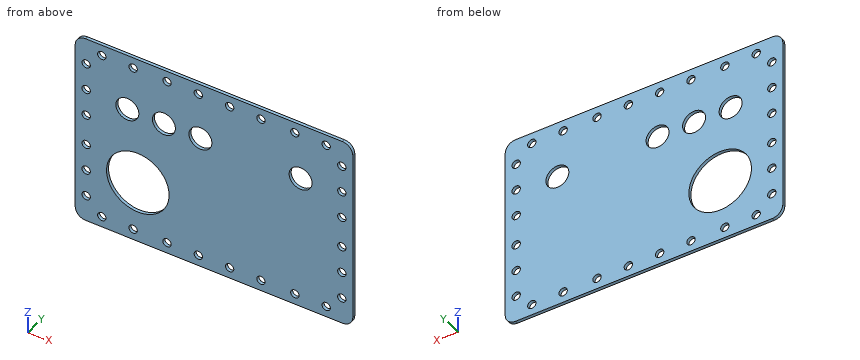
from build123d import *

# Parameters (mm, degrees)
SKETCH1_W           = 266
SKETCH1_H           = 186
BOSS_EXTRUDE1_DEPTH = 3
FILLET1_R           = 10
SKETCH2_R           = 4
SKETCH2_R_2         = 30
SKETCH2_R_3         = 11
CUT_EXTRUDE1_DEPTH  = 163.317589928


with BuildPart() as part:
    # Sketch1 → Boss-Extrude1 (new body)
    with BuildSketch(Plane(origin=(0, 0, 0), x_dir=(1, 0, 0), z_dir=(0, 1, 0))):
        Rectangle(SKETCH1_W, SKETCH1_H)
    extrude(amount=BOSS_EXTRUDE1_DEPTH)

    # Fillet1
    fillet1_edges = [part.edges().sort_by_distance(p)[0] for p in [
        (-133, 1.5, -93),
        (133, 1.5, -93),
        (133, 1.5, 93),
        (-133, 1.5, 93),
    ]]
    fillet(fillet1_edges, radius=FILLET1_R)

    # Sketch2 → Cut-Extrude1 (cut, through all)
    with BuildSketch(Plane(origin=(0, 3, 0), x_dir=(1, 0, 0), z_dir=(0, 1, 0))):
        with Locations(Location((-122.5, -15, 0), (0, 0, 270))):
            Circle(SKETCH2_R)
        with Locations(Location((-122.5, -41.25, 0), (0, 0, 270))):
            Circle(SKETCH2_R)
        with Locations(Location((-122.5, -67.5, 0), (0, 0, 270))):
            Circle(SKETCH2_R)
        with Locations(Location((-107.5, -82.5, 0), (0, 0, 270))):
            Circle(SKETCH2_R)
        with Locations(Location((-77.5, -82.5, 0), (0, 0, 270))):
            Circle(SKETCH2_R)
        with Locations(Location((-45, -82.5, 0), (0, 0, 270))):
            Circle(SKETCH2_R)
        with Locations(Location((-15, -82.5, 0), (0, 0, 270))):
            Circle(SKETCH2_R)
        with Locations(Location((-15, 82.5, 0), (0, 0, 90))):
            Circle(SKETCH2_R)
        with Locations(Location((-45, 82.5, 0), (0, 0, 90))):
            Circle(SKETCH2_R)
        with Locations(Location((-77.5, 82.5, 0), (0, 0, 90))):
            Circle(SKETCH2_R)
        with Locations(Location((-107.5, 82.5, 0), (0, 0, 90))):
            Circle(SKETCH2_R)
        with Locations(Location((-122.5, 67.5, 0), (0, 0, 90))):
            Circle(SKETCH2_R)
        with Locations(Location((-122.5, 41.25, 0), (0, 0, 90))):
            Circle(SKETCH2_R)
        with Locations(Location((-122.5, 15, 0), (0, 0, 90))):
            Circle(SKETCH2_R)
        with Locations(Location((15, -82.5, 0), (0, 0, 90))):
            Circle(SKETCH2_R)
        with Locations(Location((107.5, -82.5, 0), (0, 0, 90))):
            Circle(SKETCH2_R)
        with Locations(Location((122.5, -67.5, 0), (0, 0, 90))):
            Circle(SKETCH2_R)
        with Locations(Location((122.5, -41.25, 0), (0, 0, 90))):
            Circle(SKETCH2_R)
        with Locations(Location((122.5, -15, 0), (0, 0, 90))):
            Circle(SKETCH2_R)
        with Locations(Location((122.5, 15, 0), (0, 0, 270))):
            Circle(SKETCH2_R)
        with Locations(Location((122.5, 41.25, 0), (0, 0, 270))):
            Circle(SKETCH2_R)
        with Locations(Location((122.5, 67.5, 0), (0, 0, 270))):
            Circle(SKETCH2_R)
        with Locations(Location((107.5, 82.5, 0), (0, 0, 270))):
            Circle(SKETCH2_R)
        with Locations(Location((77.5, 82.5, 0), (0, 0, 270))):
            Circle(SKETCH2_R)
        with Locations(Location((45, 82.5, 0), (0, 0, 270))):
            Circle(SKETCH2_R)
        with Locations(Location((15, 82.5, 0), (0, 0, 270))):
            Circle(SKETCH2_R)
        with Locations(Location((-73, 33, 0), (0, 0, 270))):
            Circle(SKETCH2_R_2)
        with Locations(Location((83, -38, 0), (0, 0, 270))):
            Circle(SKETCH2_R_3)
        with Locations(Location((-83, -38, 0), (0, 0, 270))):
            Circle(SKETCH2_R_3)
        with Locations(Location((-48, -38, 0), (0, 0, 270))):
            Circle(SKETCH2_R_3)
        with Locations(Location((-13, -38, 0), (0, 0, 270))):
            Circle(SKETCH2_R_3)
        with Locations(Location((45, -82.5, 0), (0, 0, 90))):
            Circle(SKETCH2_R)
        with Locations(Location((77.5, -82.5, 0), (0, 0, 90))):
            Circle(SKETCH2_R)
    extrude(amount=-CUT_EXTRUDE1_DEPTH, mode=Mode.SUBTRACT)


solid = part.part
Geometry check sheet. Reference: the model listing, model coordinates, mm. Round coordinates to 2 decimals unless told otherwise and drop trailing zeros. Write each loop counter-clockwise with the first axis right and the second up, starting at its lowest first coordinate (ties: lowest second). Pieces come first, ordered by that corner, then holes.
Item 1: Go/stop test with flat-tipped pins: pin 1 Ø13 at (x, z) = (-15, -82.5) entering from -Y; pin 2 Ø5 at (x, z) = (-122.5, -67.5) entering from +Y. Record where each tip stops, or that it passes through.
Determined:
pin 1: stops at y = 0
pin 2: passes through
Item 2: Section check D-D (y = 1.1). Give the number of separate pieces and of enclosed holes in the cut face, plus the area to 3 significant figures.
Determined:
separate pieces: 1
enclosed holes: 33
area: 43,600 mm2
Item 3: Section check A-A (x = 15). Record the boundary of the cut face in (y, z).
Determined:
outline: (0, -93) - (3, -93) - (3, -86.5) - (0, -86.5) - close; (0, -78.5) - (3, -78.5) - (3, 78.5) - (0, 78.5) - close; (0, 86.5) - (3, 86.5) - (3, 93) - (0, 93) - close
Item 4: Section check C-C (z = -67.5). Record the boundary of the cut face in (x, y), plus the area to 3 significant figures.
Determined:
outline: (-133, 0) - (-126.5, 0) - (-126.5, 3) - (-133, 3) - close; (-118.5, 0) - (118.5, 0) - (118.5, 3) - (-118.5, 3) - close; (126.5, 0) - (133, 0) - (133, 3) - (126.5, 3) - close
area: 750 mm2
Item 5: Material ranges on line 1 along X through (y, z) = (1.05, -67.5); line 2 along X through (y, z) = (2.35, 37); line 3 along X through (y, z) = (1.75, -15), recorded low to high.
Determined:
line 1: x = -133 to -126.5, -118.5 to 118.5, 126.5 to 133
line 2: x = -133 to -93.95, -72.05 to -58.95, -37.05 to -23.95, -2.05 to 72.05, 93.95 to 133
line 3: x = -133 to -126.5, -118.5 to -97, -49 to 118.5, 126.5 to 133
Item 6: Section check B-B (z = -33). Record the boundary of the cut face in (x, y).
Determined:
outline: (-133, 0) - (-103, 0) - (-103, 3) - (-133, 3) - close; (-43, 0) - (133, 0) - (133, 3) - (-43, 3) - close
